```python
from build123d import *

# Parameters (mm, degrees)
SKETCH_1_W                  = 31
SKETCH_1_H                  = 2
SKETCH_6_R                  = 22.5
SKETCH_6_R_2                = 12
EXTRUDE_1_DEPTH             = 4
SKETCH_8_R                  = 12
SKETCH_8_R_2                = 10
EXTRUDE_3_DEPTH             = 10
SKETCH_9_R                  = 12
EXTRUDE_5_DEPTH             = 10
SKETCH_18_R                 = 10
CUT_EXTRUDE_1_DEPTH         = 46
SKETCH_17_W                 = 1.65
SKETCH_17_H                 = 51
HOLE_WIZARD_M4_1_AT_2_COUNT = 2
HOLE_WIZARD_M4_1_AT_2_PITCH = 25.455844123
HOLE_WIZARD_M4_1_AT_3_COUNT = 2
HOLE_WIZARD_M4_1_AT_3_PITCH = 36
HOLE_WIZARD_M4_1_AT_4_COUNT = 2
HOLE_WIZARD_M4_1_AT_4_PITCH = 25.455844123
SKETCH_12_W                 = 1
SKETCH_12_H                 = 2
CUT_EXTRUDE_START           = -10
SKETCH_19_R                 = 12
SKETCH_19_R_2               = 11
CUT_EXTRUDE_3_DEPTH         = 10
SKETCH_20_W                 = 2.76
SKETCH_20_H                 = 2.86
FILLET_1_R                  = 0.2
CHAMFER_1_SIZE              = 0.3
CHAMFER_2_SIZE              = 0.3
SKETCH_21_R                 = 12
SKETCH_21_R_2               = 11
EXTRUDE_6_DEPTH             = 10


with BuildPart() as part:
    # Sketch 1 → Revolve 1 (revolve)
    with BuildSketch(Plane.XY, mode=Mode.PRIVATE) as revolve_1_sk:
        with Locations((4.5, 11)):
            Rectangle(SKETCH_1_W, SKETCH_1_H)
    revolve(revolve_1_sk.sketch.rotate(Axis((-11, 0, 0), (1, 0, 0)), 90), axis=Axis((-11, 0, 0), (1, 0, 0)))

    # Sketch 6 → Extrude 1 (add)
    with BuildSketch(Plane.ZY.offset(11)):
        Circle(SKETCH_6_R)
        Circle(SKETCH_6_R_2, mode=Mode.SUBTRACT)
    extrude(amount=-EXTRUDE_1_DEPTH)

    # Sketch 8 → Extrude 3 (add)
    with BuildSketch(Plane(origin=(20, 0, 0), x_dir=(0, 0, -1), z_dir=(1, 0, 0))):
        with Locations(Location((0, 0, 0), (0, 0, 180))):
            Circle(SKETCH_8_R)
        with Locations(Location((0, 0, 0), (0, 0, 180))):
            Circle(SKETCH_8_R_2, mode=Mode.SUBTRACT)
    extrude(amount=EXTRUDE_3_DEPTH)

    # Sketch 17 → Hole Wizard M4 _1 (revolve, cut)
    with BuildSketch(Plane(origin=(-11, 18, 0), x_dir=(0, 0, 1), z_dir=(0, 1, 0))):
        with Locations((0.825, 25.5)):
            Rectangle(SKETCH_17_W, SKETCH_17_H)
    hole_wizard_m4_1 = revolve(axis=Axis((-17.35, 18, 0), (1, 0, 0)), mode=Mode.SUBTRACT)

    # Hole Wizard M4 _1 at 2: Hole Wizard M4 _1 ×2
    with Locations(*[Vector(0, -0.7071067811865476, 0.7071067811865476) * (i * HOLE_WIZARD_M4_1_AT_2_PITCH) for i in range(1, HOLE_WIZARD_M4_1_AT_2_COUNT)]):
        add(hole_wizard_m4_1, mode=Mode.SUBTRACT)

    # Hole Wizard M4 _1 at 3: Hole Wizard M4 _1 ×2
    with Locations(*[(0, -i * HOLE_WIZARD_M4_1_AT_3_PITCH, 0) for i in range(1, HOLE_WIZARD_M4_1_AT_3_COUNT)]):
        add(hole_wizard_m4_1, mode=Mode.SUBTRACT)

    # Hole Wizard M4 _1 at 4: Hole Wizard M4 _1 ×2
    with Locations(*[Vector(0, -0.7071067811865477, -0.7071067811865475) * (i * HOLE_WIZARD_M4_1_AT_4_PITCH) for i in range(1, HOLE_WIZARD_M4_1_AT_4_COUNT)]):
        add(hole_wizard_m4_1, mode=Mode.SUBTRACT)

    # Sketch 20 → Cut-Revolve 3 (revolve, cut)
    with BuildSketch(Plane(origin=(0, 0, 0), x_dir=(1, 0, 0), z_dir=(0, 1, 0)), mode=Mode.PRIVATE) as cut_revolve_3_sk:
        with Locations((-10.62, 13.7)):
            Rectangle(SKETCH_20_W, SKETCH_20_H)
    revolve(cut_revolve_3_sk.sketch.rotate(Axis((0, 0, 0), (-1, 0, 0)), 180), axis=Axis((0, 0, 0), (-1, 0, 0)), mode=Mode.SUBTRACT)

    # Fillet 1
    fillet_1_edges = [part.edges().sort_by_distance(p)[0] for p in [
        (-9.24, 0, -12.27),
        (-9.24, 0, -15.13),
    ]]
    fillet(fillet_1_edges, radius=FILLET_1_R)

    # Chamfer 1
    chamfer_1_edges = [part.edges().sort_by_distance(p)[0] for p in [
        (-11, 0, -15.13),
    ]]
    chamfer(chamfer_1_edges, length=CHAMFER_1_SIZE)

    # Chamfer 2
    chamfer_2_edges = [part.edges().sort_by_distance(p)[0] for p in [
        (-11, 0, -12.27),
    ]]
    chamfer(chamfer_2_edges, length=CHAMFER_2_SIZE)



with BuildPart() as body_2:
    # Sketch 9 → Extrude 5 (new body)
    with BuildSketch(Plane(origin=(30, 0, 0), x_dir=(0, 0, -1), z_dir=(1, 0, 0))):
        Circle(SKETCH_9_R)
    extrude(amount=EXTRUDE_5_DEPTH)

    # Sketch 18 → Cut-Extrude 1 (cut)
    with BuildSketch(Plane(origin=(-7, 0, 0), x_dir=(0, 0, -1), z_dir=(1, 0, 0))):
        Circle(SKETCH_18_R)
    extrude(amount=CUT_EXTRUDE_1_DEPTH, mode=Mode.SUBTRACT)

    # Sketch 12 → Cut-Revolve 2 (revolve, cut)
    with BuildSketch(Plane.XY, mode=Mode.PRIVATE) as cut_revolve_2_sk:
        with Locations((33.5, -12)):
            Rectangle(SKETCH_12_W, SKETCH_12_H)
        with Locations((31.5, -12)):
            Rectangle(SKETCH_12_W, SKETCH_12_H)
        with Locations((35.5, -12)):
            Rectangle(SKETCH_12_W, SKETCH_12_H)
        with Locations((37.5, -12)):
            Rectangle(SKETCH_12_W, SKETCH_12_H)
        with Locations((39.5, -12)):
            Rectangle(SKETCH_12_W, SKETCH_12_H)
    revolve(cut_revolve_2_sk.sketch.rotate(Axis((0, 0, 0), (1, 0, 0)), 270), axis=Axis((0, 0, 0), (1, 0, 0)), mode=Mode.SUBTRACT)

    # Sketch 19 → Cut-Extrude 3 (cut)
    with BuildSketch(Plane(origin=(40, 0, 0), x_dir=(0, 0, -1), z_dir=(1, 0, 0)).offset(CUT_EXTRUDE_START)):
        with Locations(Location((0, 0, 0), (0, 0, 180))):
            Circle(SKETCH_19_R)
        with Locations(Location((0, 0, 0), (0, 0, 180))):
            Circle(SKETCH_19_R_2, mode=Mode.SUBTRACT)
    extrude(amount=CUT_EXTRUDE_3_DEPTH, mode=Mode.SUBTRACT)


with BuildPart() as part_1:
    add(part.part)

    add(body_2.part)  # Extrude 6 merges body 2
    # Sketch 21 → Extrude 6 (add)
    with BuildSketch(Plane(origin=(30, 0, 0), x_dir=(0, 0, -1), z_dir=(1, 0, 0))):
        with Locations(Location((0, 0, 0), (0, 0, 180))):
            Circle(SKETCH_21_R)
        Circle(SKETCH_21_R_2, mode=Mode.SUBTRACT)
    extrude(amount=EXTRUDE_6_DEPTH)


solid = part_1.part
```
CAD build for the part. Positions are in the model's coordinates, mm. A direction names the side the tool comes from. Round coordinates to 2 decimals unless told otherwise and drop trailing zeros. Loops run counter-clockwise (first coordinate to the right, second up) from the corner with the lowest first, then second, coordinate; pieces in that order, holes last. Notation, with made-up numbers: M -30.75,31.25 L 28.25,31.25 A29 cw 28.25,65.25 Z; hole C 10,2 d10. An arc over 180 degrees is marked long. Return JSON: item names as keys, results as strings. Group by question number.
(1) Wall check: probe 1 along Y at (x, z) = (33.5, 0.5); probe 2 along X at (y, z) = (3.5, 19.5); probe 3 along Z at (x, y) = (-4, -6.5). Give the ranges that are in metal, low to high. Write a range as [from, to].
(2) Saw through at A-A, the plane z = 18. List the corners of the cut face in (x, y), and give its area (3 significant figures).
(3) Mould opens along Y. For faces 1 (the cylindrical face through (-8.972, -19.636, -0.215)), 2 (the flat face through (40, 0, 0)), 3 (the cylindrical face through (-9.028, -19.961, 10.382)) say: +Y half, -Y half, draft (parallel to the pull), parting line (faces both ways), or undercut.
(4) Drop flat-ended pins along their axis: P1, Ø3, axis at x = 26.5, z = -14.5, coming from the +Y side; P2, Ø1.5, axis at x = 14.5, z = 9, coming from the -Y side; P3, Ø4, axis at y = -7, z = -16.5, coming from the +X side; P4, Ø18, axis at y = 0, z = 0, coming from the -X side. Give the stop position or say it passes through.
(5) Saw through at C-C, the plane y = 0. Give the number of separate pieces and of enclosed holes in the cut face, and give its area (3 significant figures).
(6) Tool access for faces 4 (the flat face through (-7, -10, 10)), 5 (the cylindrical face through (-10.061, 0.665, -15.115)), 6 (the cylindrical face through (-8.97, 1, -19.31)): list every direction of +Z, -Z, +X, -X, +Y, -Y with a clear straight run to the whole face (end or side of a thin tool).
Answer list:
{
 "1": {"probe 1": "[-11.99, -9.99], [9.99, 11.99]", "probe 2": "[-11, -7]", "probe 3": "[-10.09, -7.6], [7.6, 10.09]"},
 "2": {"outline": "M -11,-13.5 L -7,-13.5 L -7,-1.65 L -11,-1.65 Z; M -11,1.65 L -7,1.65 L -7,13.5 L -11,13.5 Z", "area": "94.8 mm2"},
 "3": {"face 1": "undercut", "face 2": "draft", "face 3": "parting line"},
 "4": {"P1": "through", "P2": "y = -8.71", "P3": "x = -7", "P4": "x = 39"},
 "5": {"separate pieces": "3", "enclosed holes": "0", "area": "271 mm2"},
 "6": {"face 4": "+X", "face 5": "-X", "face 6": "+X, -X"}
}
